For this review, take the finished solid that the model builds, in its own axes (mm). Face numbers are marked on the shaded views. Give positions to 0.01 mm unless a question says otherwise; leave off trailing zeros. Order: outer loops, then holes, each group sorted by start corner. A loop starts at its lowest first (then second) coordinate and runs counter-clockwise, first axis right, second up. Notation, with made-up numbers: (-5.75, 3) - (49.25, 3) arc R20 ccw to (49.25, 13) - close; hole circle Ø5 at (2.25, -38). An arc over 180 degrees is marked (long way). One line per item, written item: value.
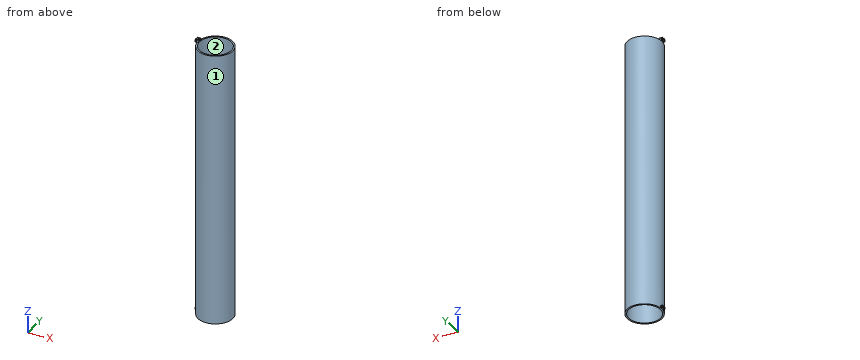
```python
from build123d import *

# Parameters (mm, degrees)
SKETCH1_R               = 22
SKETCH1_R_2             = 20
BOSS_EXTRUDE1_DEPTH     = 350
BOSS_EXTRUDE2_DEPTH     = 3
CUT_EXTRUDE1_DEPTH      = 352.746002109
CUT_EXTRUDE1_DEPTH_BACK = 352.746002109
SKETCH3_R               = 1
SKETCH4_W               = 2.837375188
SKETCH4_H               = 2.5
SKETCH4_W_2             = 2.705505282
SKETCH4_H_2             = 0.5
BOSS_EXTRUDE3_DEPTH     = 3
CUT_EXTRUDE2_DEPTH      = 352.746002109
CUT_EXTRUDE2_DEPTH_BACK = 352.746002109
SKETCH5_R               = 1
CUT_EXTRUDE3_START      = -3
SKETCH6_R               = 22
CUT_EXTRUDE3_DEPTH      = 3
SKETCH7_W               = 3
SKETCH7_H               = 6
BOSS_EXTRUDE4_DEPTH     = 4.4
CUT_EXTRUDE4_DEPTH      = 352.746002109
CUT_EXTRUDE4_DEPTH_BACK = 352.746002109
SKETCH8_R               = 1
SKETCH9_W               = 3
SKETCH9_H               = 1.25
CUT_EXTRUDE5_DEPTH      = 4.4


with BuildPart() as part:
    # Sketch1 → Boss-Extrude1 (new body)
    with BuildSketch(Plane.XY):
        Circle(SKETCH1_R)
        Circle(SKETCH1_R_2, mode=Mode.SUBTRACT)
    extrude(amount=BOSS_EXTRUDE1_DEPTH)

    # Sketch2 → Boss-Extrude2 (add)
    with BuildSketch(Plane(origin=(0, 0, 0), x_dir=(-1, 0, 0), z_dir=(0, 0, -1))):
        with BuildLine():
            Line((24.5, 3), (21.794494718, 3))
            ThreePointArc((21.794494718, 3), (21.827425588, 2.750180393), (21.857492994, 2.5))
            Line((21.857492994, 2.5), (24.5, 2.5))
            Line((24.5, 2.5), (24.5, 3))
        make_face()
        with BuildLine():
            Line((24.5, 1.25), (21.96445993, 1.25))
            ThreePointArc((21.96445993, 1.25), (21.991113188, 0.625252568), (22, 0))
            ThreePointArc((22, 0), (21.991113188, -0.625252568), (21.96445993, -1.25))
            Line((21.96445993, -1.25), (24.5, -1.25))
            Line((24.5, -1.25), (24.5, 1.25))
        make_face()
        with BuildLine():
            ThreePointArc((21.857492994, -2.5), (21.827425588, -2.750180393), (21.794494718, -3))
            Line((21.794494718, -3), (24.5, -3))
            Line((24.5, -3), (24.5, -2.5))
            Line((24.5, -2.5), (21.857492994, -2.5))
        make_face()
    extrude(amount=-BOSS_EXTRUDE2_DEPTH)

    # Sketch3 → Cut-Extrude1 (cut, two sides: drawn at the far end of the back side and taken through both)
    with BuildSketch(Plane(origin=(0, 3, 0), x_dir=(1, 0, 0), z_dir=(0, 1, 0)).offset(-CUT_EXTRUDE1_DEPTH_BACK)):
        with Locations(Location((-23.147247359, -1.5, 0), (0, 0, 180))):
            Circle(SKETCH3_R)
    extrude(amount=CUT_EXTRUDE1_DEPTH + CUT_EXTRUDE1_DEPTH_BACK, mode=Mode.SUBTRACT)

    # Sketch4 → Boss-Extrude3 (add)
    with BuildSketch(Plane.XY.offset(350)):
        with Locations((-23.081312406, 0)):
            Rectangle(SKETCH4_W, SKETCH4_H)
        with Locations((-23.147247359, 2.75)):
            Rectangle(SKETCH4_W_2, SKETCH4_H_2)
        with Locations((-23.147247359, -2.75)):
            Rectangle(SKETCH4_W_2, SKETCH4_H_2)
    extrude(amount=-BOSS_EXTRUDE3_DEPTH)

    # Sketch5 → Cut-Extrude2 (cut, two sides: drawn at the far end of the back side and taken through both)
    with BuildSketch(Plane(origin=(0, 3, 0), x_dir=(1, 0, 0), z_dir=(0, 1, 0)).offset(-CUT_EXTRUDE2_DEPTH_BACK)):
        with Locations(Location((-23.147247359, -348.5, 0), (0, 0, 270))):
            Circle(SKETCH5_R)
    extrude(amount=CUT_EXTRUDE2_DEPTH + CUT_EXTRUDE2_DEPTH_BACK, mode=Mode.SUBTRACT)

    # Sketch6 → Cut-Extrude3 (cut)
    with BuildSketch(Plane.XY.offset(350).offset(CUT_EXTRUDE3_START)):
        with Locations(Location((0, 0, 0), (0, 0, 180))):
            Circle(SKETCH6_R)
    extrude(amount=CUT_EXTRUDE3_DEPTH, mode=Mode.SUBTRACT)


with BuildPart() as cut_extrude3_piece_1:
    # of the separate pieces the step leaves, piece 1, a body of its own (cut_extrude3_pieces)
    add(part.part.solids().sort_by_distance((22, 0, 0))[0])



with BuildPart() as cut_extrude3_piece_2:
    # of the separate pieces the step leaves, piece 2, a body of its own (cut_extrude3_pieces)
    add(part.part.solids().sort_by_distance((-24.5, 1.25, 347))[0])


with BuildPart() as cut_extrude3_piece_3:
    # of the separate pieces the step leaves, piece 3, a body of its own (cut_extrude3_pieces)
    add(part.part.solids().sort_by_distance((-24.5, -2.5, 347))[0])


with BuildPart() as cut_extrude3_piece_4:
    # of the separate pieces the step leaves, piece 4, a body of its own (cut_extrude3_pieces)
    add(part.part.solids().sort_by_distance((-24.5, 2.5, 347))[0])


with BuildPart() as cut_extrude3_piece_1_1:
    add(cut_extrude3_piece_1.part)

    add(cut_extrude3_piece_2.part)  # Boss-Extrude4 merges Cut-Extrude3 piece 2

    add(cut_extrude3_piece_3.part)  # Boss-Extrude4 merges Cut-Extrude3 piece 3

    add(cut_extrude3_piece_4.part)  # Boss-Extrude4 merges Cut-Extrude3 piece 4
    # Sketch7 → Boss-Extrude4 (add)
    with BuildSketch(Plane.ZY.offset(24.5)):
        with Locations((348.5, 0)):
            Rectangle(SKETCH7_W, SKETCH7_H)
    extrude(amount=-BOSS_EXTRUDE4_DEPTH)

    # Sketch8 → Cut-Extrude4 (cut, two sides: drawn at the far end of the back side and taken through both)
    with BuildSketch(Plane(origin=(0, 3, 0), x_dir=(1, 0, 0), z_dir=(0, 1, 0)).offset(-CUT_EXTRUDE4_DEPTH_BACK)):
        with Locations(Location((-23.25, -348.5, 0), (0, 0, 270))):
            Circle(SKETCH8_R)
    extrude(amount=CUT_EXTRUDE4_DEPTH + CUT_EXTRUDE4_DEPTH_BACK, mode=Mode.SUBTRACT)

    # Sketch9 → Cut-Extrude5 (cut)
    with BuildSketch(Plane.ZY.offset(24.5)):
        with Locations((348.5, 1.875)):
            Rectangle(SKETCH9_W, SKETCH9_H)
        with Locations((348.5, -1.875)):
            Rectangle(SKETCH9_W, SKETCH9_H)
    extrude(amount=-CUT_EXTRUDE5_DEPTH, mode=Mode.SUBTRACT)


solid = cut_extrude3_piece_1_1.part
```
(1) For P1, Ø0.9, axis at x = -22.5, z = 348, coming from the +Y side; P2, Ø12, axis at x = 4, y = -8, coming from the -Z side; P3, Ø1.4, axis at x = -23, z = 2, coming from the -Y side; P4, Ø5, axis at y = -15.5, z = 73.5, coming from the +X side, all flat-tipped, find the tip position at first contact; note any pin that passes through.
Answers below:
P1: stops at y = 3
P2: passes through
P3: stops at y = -3
P4: stops at x = 17.75
(2) Take a section at B-B (y = -7.5). Write out the cut boundary in (x, z), then the cut area to 3 significant figures.
Answers below:
outline: (-20.68, 0) - (-18.54, 0) - (-18.54, 347) - (-20.68, 347) - close; (18.54, 0) - (20.68, 0) - (20.68, 347) - (18.54, 347) - close
area: 1,490 mm^2
(3) Take a section at A-A (x = 0). Write out the cut boundary in (y, z).
Answers below:
outline: (-22, 0) - (-20, 0) - (-20, 347) - (-22, 347) - close; (20, 0) - (22, 0) - (22, 347) - (20, 347) - close
(4) Draft analysis for pull direction X (two halves, no side actions). For the marked faces 1 and 2, state which applies: pulls with the +X half, pulls with the -X half, needs draft (parallel to the pull), parting line crosses it, or undercut.
Answers below:
face 1: parting line crosses it
face 2: undercut
(5) Wall thickness on line 1 (Z direction, x = -23.25, y = 2.7); line 2 (Y direction, x = -1.5, z = 300); line 3 (X direction, y = 2.8, z = 348.5): over which ranges is each line inside the solid? List them lowest first. Write a range as from..to.
Answers below:
line 1: z = 0..0.51, 2.49..3, 347..347.5, 349.5..350
line 2: y = -21.95..-19.94, 19.94..21.95
line 3: x = -24.5..-24.25, -22.25..-20.1
(6) Take a section at C-C (z = 155.5). Write out the cut boundary in (x, y).
Answers below:
outline: circle Ø44 at (0, 0); hole circle Ø40 at (0, 0)
